Design review of the part shown in the three views and the two pictorial views. Dimensions are in mm from the part's minimum x, y and z. A direction names the side the tool comes from. Coordinates: 2 decimals unless noted, no trailing zeros. Order: outer loops, then holes, each group sorted by start corner. A loop starts at its lowest first (then second) coordinate and runs counter-clockwise, first axis right, second up. Notation, with made-up numbers: (74, 77.5) -> (95, 77.5) arc R13 cw to (95, 98.5) -> close; hole circle Ø3 at (21, -6). An arc over 180 degrees is marked (long way). Answer as a JSON object with one key per item and string values. Group by question number.
1) Wall thickness on L1, parallel to Y at x = 18.5, z = 70; L2, parallel to Y at x = 167, z = 62.55; L3, parallel to Z at x = 118, y = 40.5: over which ranges is each line inside the solid? List them lowest first.
2) Machinability: for the marked faces 1, 2, 3 and 4, which of the approach directions +Z, -Z, +X, -X, +Y, -Y give a long, thin tool a straight path to every point of the face, cutting with its end or side? Answer none if there is none.
3) Draft analysis for pull direction Z (two halves, no side actions). For the marked faces 5, 6 and 7, state which applies: +Z half, -Z half, draft (parallel to the pull), parting line (faces both ways), or undercut.
4) Add section A-A, the plane z = 38.5. Write out the cut boundary in (x, y), then the cut area to 3 significant figures.
5) For pin 1 (4 mm diameter, centred on y = 20.5, z = 70, fed in from +X); pin 2 (8 mm diameter, centred on y = 16, z = 36, fed in from -X); pin 3 (5 mm diameter, centred on x = 20, z = 69.5, fed in from +Y); pin 4 (12 mm diameter, centred on y = 5.5, z = 48.5, fed in from +X), all flat-tipped, find the tip position at first contact; note any pin that passes through.
6) Add section B-B, the plane x = 239.5. Write out the cut boundary in (y, z), then the cut area to 3 significant figures.
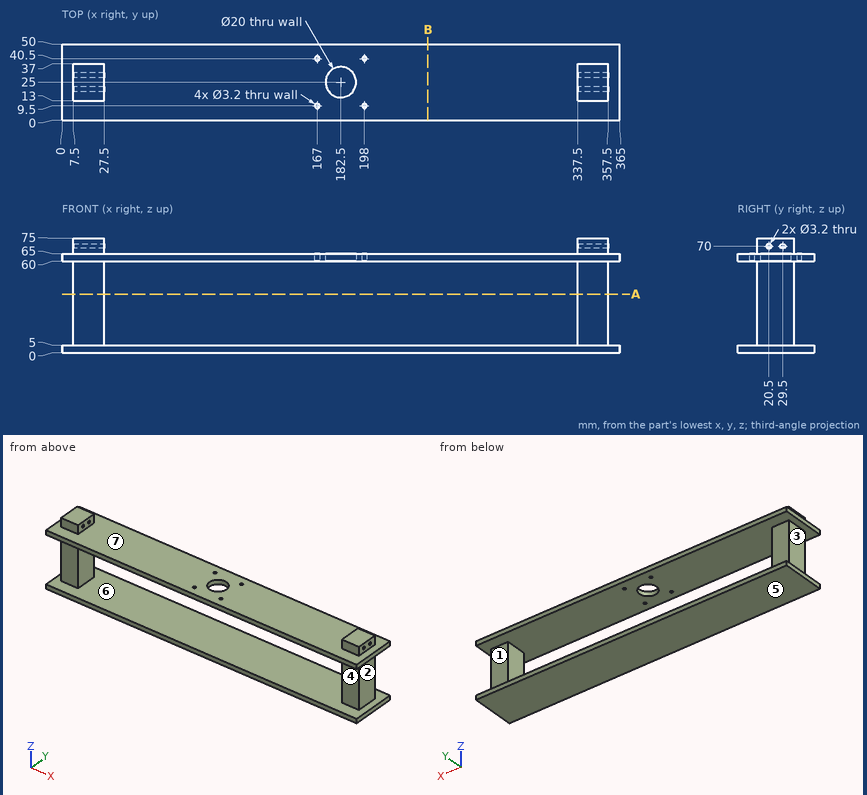
Output values:
{
 "1": {"L1": "y = 13 to 18.9, 22.1 to 27.9, 31.1 to 37", "L2": "y = 0 to 7.9, 11.1 to 38.9, 42.1 to 50", "L3": "z = 0 to 5, 60 to 65"},
 "2": {"face 1": "+X, -X, +Y", "face 2": "+X, +Y, -Y", "face 3": "-X, +Y, -Y", "face 4": "+X, -X, -Y"},
 "3": {"face 5": "-Z half", "face 6": "undercut", "face 7": "+Z half"},
 "4": {"outline": "(7.5, 13) -> (27.5, 13) -> (27.5, 37) -> (7.5, 37) -> close; (337.5, 13) -> (357.5, 13) -> (357.5, 37) -> (337.5, 37) -> close", "area": "960 mm²"},
 "5": {"pin 1": "stops at x = 357.5", "pin 2": "stops at x = 7.5", "pin 3": "stops at y = 37", "pin 4": "passes through"},
 "6": {"outline": "(0, 0) -> (50, 0) -> (50, 5) -> (0, 5) -> close; (0, 60) -> (50, 60) -> (50, 65) -> (0, 65) -> close", "area": "500 mm²"}
}
